Here's how the part is built. I have some questions about the finished solid (model axes, mm). A direction names the side the tool comes from. Coordinates: 2 decimals unless noted, no trailing zeros. Order: outer loops, then holes, each group sorted by start corner. A loop starts at its lowest first (then second) coordinate and runs counter-clockwise, first axis right, second up. Notation, with made-up numbers: (-18.5, -29.5) - (20.5, -29.5) arc R30 ccw to (20.5, 6.5) - close; hole circle Ø4 at (33, 77). An arc over 180 degrees is marked (long way). Answer in a Markdown table with one row per item. Add a question column.
Item 1: I want a section at A-A (x = 35.5). Please give me the cut outline in (y, z).
Item 2: Thinking about a two-plate mould opening in X: for faces 1 (the cylindrical face through (22.05, 9.4, -0.57)), 2 (the flat face through (4, 7.8, -4)), which applies, +X half, -X half, draft (parallel to the pull), parting line (faces both ways), or undercut?
Item 3: Will these pins go through, and if not, where does the flat tip stop? pin 1 Ø4 at (y, z) = (5, -5) entering from +X; pin 2 Ø0.7 at (x, y) = (35, 8.5) entering from +Z; pin 3 Ø1.7 at (x, y) = (11.5, 4.5) entering from +Z; pin 4 Ø2 at (x, z) = (35.5, -5) entering from -Y.
Item 4: I want a section at D-D (x = 10). Please give me the cut outline in (y, z), plus the area to 3 significant figures.
Item 5: If I drill on line 1 along X through (y, z) = (2, -5); line 2 along Y through (x, z) = (1.5, -5); line 3 along Z through (x, y) = (1.4, 5), over which ranges is the centre line in solid material (lowest first)? Write a range as from..to.
Item 6: I want a section at C-C (x = 40). Please give me the cut outline in (y, z).
Item 7: On a 3-axis mill with a long thin cutter (end or side, diameter ignored), from which of +Z, -Z, +X, -X, +Y, -Y can I reach the whole of each face in a straight line? I mean faces 3 (the flat face through (5.3, 5, -4)), 4 (the flat face through (10.414, 8.915, -3.58)), 5 (the flat face through (21, 4, 0)). Say none if no direction works.
Item 8: I want a section at B-B (z = -1.5). Please give me the cut outline in (x, y).
```python
from build123d import *

# Parameters (mm, degrees)
SKETCH1_W           = 43.5
SKETCH1_H           = 10
BOSS_EXTRUDE1_DEPTH = 10
SKETCH2_R           = 1.25
CUT_EXTRUDE1_DEPTH  = 10
SKETCH3_R           = 1.25
CUT_EXTRUDE2_DEPTH  = 10
SKETCH4_R           = 1.25
CUT_EXTRUDE3_DEPTH  = 4
CUT_EXTRUDE4_START  = -4
SKETCH5_R           = 1.25
CUT_EXTRUDE4_DEPTH  = 4
CUT_EXTRUDE5_DEPTH  = 2.2
CUT_EXTRUDE6_DEPTH  = 2.2
CUT_EXTRUDE7_DEPTH  = 2.2
CUT_EXTRUDE8_DEPTH  = 2.2
SKETCH11_W          = 2.3
SKETCH11_H          = 5.6
CUT_EXTRUDE9_DEPTH  = 7.3
FILLET1_R           = 2


with BuildPart() as part:
    # Sketch1 → Boss-Extrude1 (new body)
    with BuildSketch(Plane(origin=(0, 0, 0), x_dir=(1, 0, 0), z_dir=(0, 1, 0))):
        with Locations((21.75, 5)):
            Rectangle(SKETCH1_W, SKETCH1_H)
    extrude(amount=BOSS_EXTRUDE1_DEPTH)

    # Sketch2 → Cut-Extrude1 (cut)
    with BuildSketch(Plane(origin=(0, 10, 0), x_dir=(1, 0, 0), z_dir=(0, 1, 0))):
        with Locations(Location((8, 5, 0), (0, 0, 270))):
            Circle(SKETCH2_R)
        with Locations(Location((35.5, 5, 0), (0, 0, 270))):
            Circle(SKETCH2_R)
    extrude(amount=-CUT_EXTRUDE1_DEPTH, mode=Mode.SUBTRACT)

    # Sketch3 → Cut-Extrude2 (cut)
    with BuildSketch(Plane(origin=(0, 0, -10), x_dir=(-1, 0, 0), z_dir=(0, 0, -1))):
        with Locations((-31.5, 5)):
            Circle(SKETCH3_R)
        with Locations((-12, 5)):
            Circle(SKETCH3_R)
    extrude(amount=-CUT_EXTRUDE2_DEPTH, mode=Mode.SUBTRACT)

    # Sketch4 → Cut-Extrude3 (cut)
    with BuildSketch(Plane(origin=(43.5, 0, 0), x_dir=(0, 0, -1), z_dir=(1, 0, 0))):
        with Locations((5, 5)):
            Circle(SKETCH4_R)
    extrude(amount=-CUT_EXTRUDE3_DEPTH, mode=Mode.SUBTRACT)

    # Sketch5 → Cut-Extrude4 (cut)
    with BuildSketch(Plane.ZY.offset(CUT_EXTRUDE4_START)):
        with Locations(Location((-5, 5, 0), (0, 0, 180))):
            Circle(SKETCH5_R)
    extrude(amount=CUT_EXTRUDE4_DEPTH, mode=Mode.SUBTRACT)

    # Sketch6 → Cut-Extrude5 (cut)
    with BuildSketch(Plane(origin=(0, 10, 0), x_dir=(1, 0, 0), z_dir=(0, 1, 0))):
        Polygon((9.616580754, 2.2), (11.233161507, 5), (9.616580754, 7.8), (6.383419246, 7.8), (4.766838493, 5), (6.383419246, 2.2), align=None)
    extrude(amount=-CUT_EXTRUDE5_DEPTH, mode=Mode.SUBTRACT)

    # Sketch7 → Cut-Extrude6 (cut)
    with BuildSketch(Plane(origin=(0, 10, 0), x_dir=(1, 0, 0), z_dir=(0, 1, 0))):
        Polygon((33.883419246, 7.8), (32.266838493, 5), (33.883419246, 2.2), (37.116580754, 2.2), (38.733161507, 5), (37.116580754, 7.8), align=None)
    extrude(amount=-CUT_EXTRUDE6_DEPTH, mode=Mode.SUBTRACT)

    # Sketch8 → Cut-Extrude7 (cut)
    with BuildSketch(Plane.XY):
        Polygon((10.383419246, 2.2), (13.616580754, 2.2), (15.233161507, 5), (13.616580754, 7.8), (10.383419246, 7.8), (8.766838493, 5), align=None)
    extrude(amount=-CUT_EXTRUDE7_DEPTH, mode=Mode.SUBTRACT)

    # Sketch9 → Cut-Extrude8 (cut)
    with BuildSketch(Plane.XY):
        Polygon((33.116580754, 7.8), (29.883419246, 7.8), (28.266838493, 5), (29.883419246, 2.2), (33.116580754, 2.2), (34.733161507, 5), align=None)
    extrude(amount=-CUT_EXTRUDE8_DEPTH, mode=Mode.SUBTRACT)

    # Sketch11 → Cut-Extrude9 (cut)
    with BuildSketch(Plane.XY):
        with Locations((4.15, 5)):
            Rectangle(SKETCH11_W, SKETCH11_H)
        with Locations((39.35, 5)):
            Rectangle(SKETCH11_W, SKETCH11_H)
    extrude(amount=-CUT_EXTRUDE9_DEPTH, mode=Mode.SUBTRACT)

    # Fillet1
    fillet1_edges = [part.edges().sort_by_distance(p)[0] for p in [
        (21.75, 10, 0),
    ]]
    fillet(fillet1_edges, radius=FILLET1_R)


solid = part.part
```
Values follow:
| question | item | result |
|---|---|---|
| 1 | outline | (0, -10) - (10, -10) - (10, -7.8) - (7.8, -7.8) - (7.8, -6.25) - (0, -6.25) - close; (0, -3.75) - (7.8, -3.75) - (7.8, -2.2) - (10, -2.2) - (10, -2) arc R2 ccw to (8, 0) - (0, 0) - close |
| 2 | face 1 | draft |
| 2 | face 2 | undercut |
| 3 | pin 1 | stops at x = 43.5 |
| 3 | pin 2 | stops at z = -0.01 |
| 3 | pin 3 | stops at z = -2.2 |
| 3 | pin 4 | passes through |
| 4 | outline | (0, -10) - (10, -10) - (10, -7.14) - (7.8, -7.14) - (7.8, -2.86) - (10, -2.86) - (10, -2) arc R2 ccw to (8, 0) - (7.14, 0) - (7.14, -2.2) - (2.86, -2.2) - (2.86, 0) - (0, 0) - close |
| 4 | area | 80.3 mm^2 |
| 5 | line 1 | x = 0..6.75, 9.25..34.25, 36.75..43.5 |
| 5 | line 2 | y = 0..3.75, 6.25..10 |
| 5 | line 3 | z = -10..-6.25, -3.75..0 |
| 6 | outline | (0, -10) - (10, -10) - (10, -2) arc R2 ccw to (8, 0) - (7.8, 0) - (7.8, -7.3) - (2.2, -7.3) - (2.2, 0) - (0, 0) - close |
| 7 | face 3 | +Z |
| 7 | face 4 | +Y |
| 7 | face 5 | +Z, +X, -X, +Y, -Y |
| 8 | outline | (0, 0) - (43.5, 0) - (43.5, 9.94) - (0, 9.94) - close; hole (3, 2.2) - (5.3, 2.2) - (5.3, 7.8) - (3, 7.8) - close; hole (8.77, 5) - (10.38, 2.2) - (13.62, 2.2) - (15.23, 5) - (13.62, 7.8) - (10.38, 7.8) - close; hole (28.27, 5) - (29.88, 2.2) - (33.12, 2.2) - (34.73, 5) - (33.12, 7.8) - (29.88, 7.8) - close; hole (38.2, 2.2) - (40.5, 2.2) - (40.5, 7.8) - (38.2, 7.8) - close |
